Verification items for the finished model (mm, model axes). A direction names the side the tool comes from. Coordinates: 2 decimals unless noted, no trailing zeros. Write each loop counter-clockwise with the first axis right and the second up, starting at its lowest first coordinate (ties: lowest second). Pieces come first, ordered by that corner, then holes. Notation, with made-up numbers: (58, 14) - (64, 14) arc R19 cw to (64, 43) - close; hole circle Ø5 at (71, -15). An arc over 180 degrees is marked (long way). Use one line per item in the form item = value. Start each with the question number.
(1) Sectioned sample at A-A (y = -3.75). Count the separate pieces of the cut face and the enclosed holes in it, and give its area (3 significant figures).
(2) Sectioned sample at C-C (z = 40). Record the cut outline in (x, y), and give its area (3 significant figures).
(3) Material ranges on line 1 (X direction, y = -4.75, z = 114.3) (3 decimals); line 2 (Z direction, x = 44.45, y = -4.75) (3 decimals); line 3 (X direction, y = -7, z = -2), recorded low to high. Write a range as [from, to].
(4) Tool access check on faces 1 (the flat face through (12.68, -6.26, 89.56)), 2 (the flat face through (13.537, -6.261, 39.443)). Record the directions out of +Z, -Z, +X, -X, +Y, -Y that give a thin tool (end or side, any length) a straight path to the whole face; none if there is none.
(5) Gauge pin test, flat ends, axial feed: pin 1 Ø5.5 at (x, z) = (0, 0) entering from -Y; pin 2 Ø4 at (x, y) = (6.5, -3.5) entering from +Z (3 decimals); pin 3 Ø4 at (x, y) = (4.5, -9) entering from +Z; pin 4 Ø6 at (x, y) = (34, -10) entering from +Z. Record the tip position at first contact, or that the pin passes through.
(6) Sectioned sample at B-B (z = 86). Record the cut outline in (x, y).
(7) Mould release check, pull along Z, two halves, no side actions. Record for faces 3 (the cylindrical face through (-3.588, -6.261, 103.173)), 4 (the cylindrical face through (41.52, -6.26, -1.22)), 5 (the cylindrical face through (-6.81, -6.26, -6.66)), 6 (the cylindrical face through (0.209, -6.261, 123.823)): released by +Z, released by -Z, zero draft, split by the parting line, or undercut.
from build123d import *

# Parameters (mm, degrees)
F0_R     = 3.175
F1_DEPTH = 12.7


# Not quite as in the source:
# - a feature names something its author has since deleted; it is built from what else it names


with BuildPart() as f1:
    # F0 (on Front) → F1 (new body)
    with BuildSketch(Plane.XZ):
        with BuildLine():
            Line((0, 9.525), (0, 3.175))
            ThreePointArc((0, 3.175), (2.2450640303, 2.2450640303), (3.175, 0))
            Line((3.175, 0), (9.525, 0))
            ThreePointArc((9.525, 0), (6.7351920908, 6.7351920908), (0, 9.525))
        make_face()
        with BuildLine():
            ThreePointArc((3.175, 0), (-2.2450640303, -2.2450640303), (0, 3.175))
            Line((0, 3.175), (0, 9.525))
            ThreePointArc((0, 9.525), (-6.7351920908, 6.7351920908), (-9.525, 0))
            ThreePointArc((-9.525, 0), (-6.7351920908, -6.7351920908), (0, -9.525))
            Line((0, -9.525), (0.6773435479, -9.500885786))
            ThreePointArc((0.6773435479, -9.500885786), (6.9705567315, -6.4912990883), (9.525, 0))
            Line((9.525, 0), (3.175, 0))
        make_face()
        with BuildLine():
            ThreePointArc((-9.525, 0), (-6.7351920908, 6.7351920908), (0, 9.525))
            Line((0, 9.525), (0, 47.625))
            ThreePointArc((0, 47.625), (-10.644756084, 51.722700101), (-15.7942028036, 61.9003804205))
            Line((-15.7942028036, 61.9003804205), (-9.525, 0))
        make_face()
        with BuildLine():
            Line((0, 47.625), (0, 9.525))
            ThreePointArc((0, 9.525), (6.7351920908, 6.7351920908), (9.525, 0))
            Line((9.525, 0), (36.5125, 0))
            ThreePointArc((36.5125, 0), (38.9384772185, 5.7120069047), (44.7334821429, 7.9324362036))
            Line((44.7334821429, 7.9324362036), (18.9676000005, 8.8532337108))
            ThreePointArc((18.9676000005, 8.8532337108), (13.2611998974, 11.5713591498), (11.3411865923, 17.5933818124))
            Line((11.3411865923, 17.5933818124), (15.7954255641, 61.9125))
            ThreePointArc((15.7954255641, 61.9125), (10.6492737428, 51.7267849017), (0, 47.625))
        make_face()
        with BuildLine():
            Line((36.5125, 0), (9.525, 0))
            ThreePointArc((9.525, 0), (6.9705567315, -6.4912990883), (0.6773435479, -9.500885786))
            Line((0.6773435479, -9.500885786), (44.7324052746, -7.9324746146))
            ThreePointArc((44.7324052746, -7.9324746146), (38.9380895153, -5.7116327839), (36.5125, 0))
        make_face()
        with BuildLine():
            ThreePointArc((44.7334821429, 7.9324362036), (38.9384772185, 5.7120069047), (36.5125, 0))
            ThreePointArc((36.5125, 0), (38.9380895153, -5.7116327839), (44.7324052746, -7.9324746146))
            ThreePointArc((44.7324052746, -7.9324746146), (50.1616327839, -5.5119104847), (52.3875, 0))
            ThreePointArc((52.3875, 0), (50.1620069047, 5.5115227815), (44.7334821429, 7.9324362036))
        make_face()
        with BuildLine():
            ThreePointArc((47.625, 0), (44.45, -3.175), (41.275, 0))
            ThreePointArc((41.275, 0), (44.45, 3.175), (47.625, 0))
        make_face(mode=Mode.SUBTRACT)
        with BuildLine():
            Line((0, 60.325), (0, 47.625))
            ThreePointArc((0, 47.625), (10.6492737428, 51.7267849017), (15.7954255641, 61.9125))
            ThreePointArc((15.7954255641, 61.9125), (15.8550939106, 62.7052534459), (15.875, 63.5))
            ThreePointArc((15.875, 63.5), (15.8430821396, 64.5061676396), (15.7474569047, 65.5082893304))
            ThreePointArc((15.7474569047, 65.5082893304), (10.4912828548, 75.4142187767), (0, 79.375))
            Line((0, 79.375), (0, 66.675))
            ThreePointArc((0, 66.675), (2.2450640303, 65.7450640303), (3.175, 63.5))
            ThreePointArc((3.175, 63.5), (2.2450640303, 61.2549359697), (0, 60.325))
        make_face()
        with BuildLine():
            ThreePointArc((-15.7942028036, 61.9003804205), (-10.644756084, 51.722700101), (0, 47.625))
            Line((0, 47.625), (0, 60.325))
            ThreePointArc((0, 60.325), (-3.175, 63.5), (0, 66.675))
            Line((0, 66.675), (0, 79.375))
            ThreePointArc((0, 79.375), (-10.4912828548, 75.4142187767), (-15.7474569047, 65.5082893304))
            ThreePointArc((-15.7474569047, 65.5082893304), (-15.873667691, 63.7056672947), (-15.7942028036, 61.9003804205))
        make_face()
        with BuildLine():
            Line((0, 100.0252), (0, 79.375))
            ThreePointArc((0, 79.375), (10.4912828548, 75.4142187767), (15.7474569047, 65.5082893304))
            Line((15.7474569047, 65.5082893304), (9.525, 114.3))
            ThreePointArc((9.525, 114.3), (6.7351920908, 107.5648079092), (0, 104.775))
            Line((0, 104.775), (0, 100.0252))
        make_face()
        with BuildLine():
            Line((-9.525, 114.3), (-15.7474569047, 65.5082893304))
            ThreePointArc((-15.7474569047, 65.5082893304), (-10.4912828548, 75.4142187767), (0, 79.375))
            Line((0, 79.375), (0, 100.0252))
            Line((0, 100.0252), (0, 104.775))
            ThreePointArc((0, 104.775), (-6.7351920908, 107.5648079092), (-9.525, 114.3))
        make_face()
        with Locations((-3.175, 100.0252)):
            Circle(F0_R, mode=Mode.SUBTRACT)
        with BuildLine():
            ThreePointArc((9.525, 114.3), (0, 123.825), (-9.525, 114.3))
            ThreePointArc((-9.525, 114.3), (-6.7351920908, 107.5648079092), (0, 104.775))
            ThreePointArc((0, 104.775), (6.7351920908, 107.5648079092), (9.525, 114.3))
        make_face()
        with BuildLine():
            ThreePointArc((3.175, 114.3), (2.2450640303, 112.0549359697), (0, 111.125))
            ThreePointArc((0, 111.125), (-2.2450640303, 116.5450640303), (3.175, 114.3))
        make_face(mode=Mode.SUBTRACT)
    extrude(amount=F1_DEPTH)


solid = f1.part
Answers below:
q1.separate_pieces = 1
q1.enclosed_holes = 5
q1.area = 3,770 mm2
q2.outline = (-13.58, -12.7) - (13.59, -12.7) - (13.59, 0) - (-13.58, 0) - close
q2.area = 345 mm2
q3.line_1 = [-9.525, -3.175], [3.175, 9.525]
q3.line_2 = [-7.943, -3.175], [3.175, 7.943]
q3.line_3 = [-9.31, -2.47], [2.47, 41.98], [46.92, 52.13]
q4.face_1 = +Z, +X, +Y, -Y
q4.face_2 = +X, +Y, -Y
q5.pin_1 = through
q5.pin_2 = 122.695
q5.pin_3 = 123.49
q5.pin_4 = 8.42
q6.outline = (-13.13, -12.7) - (13.13, -12.7) - (13.13, 0) - (-13.13, 0) - close
q7.face_3 = undercut
q7.face_4 = undercut
q7.face_5 = released by -Z
q7.face_6 = released by +Z
